from build123d import *

# Parameters (mm, degrees)
F0_R     = 10
F1_DEPTH = 25
F3_DEPTH = 65
F4_W     = 35
F4_H     = 5
F5_DEPTH = 15


with BuildPart() as f1:
    # F0 (on Front) → F1 (new body)
    with BuildSketch(Plane.XZ):
        Polygon((-30, 0), (30, 0), (30, 70), (15, 80), (-15, 80), (-30, 70), align=None)
        with Locations((0, 45)):
            Circle(F0_R, mode=Mode.SUBTRACT)
    extrude(amount=F1_DEPTH)

    # F2 (on face) → F3 (cut)
    with BuildSketch(Plane.XY.offset(80)):
        Polygon((-30, -25), (-15, -25), (30, -25), (30, -15), (-30, -15), align=None)
    extrude(amount=-F3_DEPTH, mode=Mode.SUBTRACT)

    # F4 (on Top) → F5 (cut)
    with BuildSketch(Plane.XY):
        with Locations((0, -22.5)):
            Rectangle(F4_W, F4_H)
    extrude(amount=F5_DEPTH, mode=Mode.SUBTRACT)


solid = f1.part
Check sheet for the modelled part. Datum: model origin and axes. Units: mm. A direction names the side the tool comes from. Round coordinates to 2 decimals unless told otherwise and drop trailing zeros. Write each loop counter-clockwise with the first axis right and the second up, starting at its lowest first coordinate (ties: lowest second). Pieces come first, ordered by that corner, then holes. Notation, with made-up numbers: (51.25, 47.25) -> (77.25, 47.25) arc R26 cw to (77.25, 85.25) -> close; hole circle Ø8 at (68.25, -0.5). An arc over 180 degrees is marked (long way). Answer as CSV lines item,"result". Start each with the question number.
1) Material ranges on line 1 (Z direction, x = 0, y = -8.5); line 2 (X direction, y = -6, z = 45); line 3 (Z direction, x = 1, y = -17.5), recorded low to high. Write a range as from..to.
2) Section check B-B on y = -5. Enter the section's corners in (x, z), and give its area (3 significant figures).
3) Section check D-D on z = 53. Enter the section's corners in (x, y).
4) Go/stop test with flat-tipped pins: P1, Ø1.5, axis at x = 6, z = 32, coming from the +Y side; P2, Ø16.5, axis at x = -1, z = 6.5, coming from the -Y side; P3, Ø4, axis at x = 18, z = 32, coming from the -Y side. Record where each tip stops, or that it passes through.
5) Section check C-C on x = 0. Enter the section's corners in (y, z).
6) Section check A-A on z = 45. Enter the section's corners in (x, y).
7) Tool access check on faces 1 (the flat face through (0, -19, 15)), 2 (the flat face through (-17.5, -23, 7)), 3 (the flat face through (0, 0, 32)). Record the directions out of +Z, -Z, +X, -X, +Y, -Y that give a thin tool (end or side, any length) a straight path to the whole face; none if there is none.
8) Release check for a two-part mould opening along Z. For faces 4 (the flat face through (30, -10, 27)), 5 (the flat face through (-22.395, -7.395, 75.07)), 6 (the flat face through (0, -12, 0)), 7 (the cylindrical face through (-2.17, -7.4, 35.24)) record: pulls with the +Z half, pulls with the -Z half, needs draft (parallel to the pull), parting line crosses it, or undercut.
Found:
1,line 1,"z = 0..35, 55..80"
1,line 2,"x = -30..-10, 10..30"
1,line 3,"z = 0..15"
2,outline,"(-30, 0) -> (30, 0) -> (30, 70) -> (15, 80) -> (-15, 80) -> (-30, 70) -> close; hole circle Ø20 at (0, 45)"
2,area,"4,340 mm^2"
3,outline,"(-30, -15) -> (-6, -15) -> (-6, 0) -> (-30, 0) -> close; (6, -15) -> (30, -15) -> (30, 0) -> (6, 0) -> close"
4,P1,"stops at y = 0"
4,P2,"stops at y = -20"
4,P3,"stops at y = -15"
5,outline,"(-20, 0) -> (0, 0) -> (0, 35) -> (-15, 35) -> (-15, 15) -> (-20, 15) -> close; (-15, 55) -> (0, 55) -> (0, 80) -> (-15, 80) -> close"
6,outline,"(-30, -15) -> (-10, -15) -> (-10, 0) -> (-30, 0) -> close; (10, -15) -> (30, -15) -> (30, 0) -> (10, 0) -> close"
7,face 1,"+Z, +X, -X, -Y"
7,face 2,"+Z, -Z, -Y"
7,face 3,"+Z, -Z, +X, -X, +Y"
8,face 4,"needs draft"
8,face 5,"pulls with the +Z half"
8,face 6,"pulls with the -Z half"
8,face 7,"undercut"
